from build123d import *

# Parameters (mm, degrees)
BASE_EXTRUDE_DEPTH = 3.048
SKETCH4_R          = 3.2385
REARRIB_DEPTH      = 3.048


with BuildPart() as part:
    # Sketch2 → Base-Extrude (new body)
    with BuildSketch(Plane(origin=(0, 0, 0), x_dir=(1, 0, 0), z_dir=(0, 1, 0))):
        with BuildLine():
            Line((0, 13.97), (7.747, 13.97))
            Line((7.747, 13.97), (7.747, 9.652))
            ThreePointArc((7.747, 9.652), (11.176, 6.223), (14.605, 9.652))
            Line((14.605, 9.652), (14.605, 13.97))
            Line((14.605, 13.97), (16.637, 13.97))
            ThreePointArc((16.637, 13.97), (19.061669153, 12.965669153), (20.066, 10.541))
            Line((20.066, 10.541), (20.066, -10.541))
            ThreePointArc((20.066, -10.541), (19.061669153, -12.965669153), (16.637, -13.97))
            Line((16.637, -13.97), (14.605, -13.97))
            Line((14.605, -13.97), (14.605, -9.398))
            ThreePointArc((14.605, -9.398), (11.176, -5.969), (7.747, -9.398))
            Line((7.747, -9.398), (7.747, -13.97))
            Line((7.747, -13.97), (0, -13.97))
            Line((0, -13.97), (0, 13.97))
        make_face()
    extrude(amount=BASE_EXTRUDE_DEPTH)

    # Sketch4 → RearRib (add)
    with BuildSketch(Plane.ZY):
        with BuildLine():
            Line((13.97, 22.352), (13.97, 0))
            Line((13.97, 0), (-13.97, 0))
            Line((-13.97, 0), (-13.97, 6.35))
            Line((-13.97, 6.35), (-0.465269586, 26.70511583))
            ThreePointArc((-0.465269586, 26.70511583), (8.369371866, 29.890677361), (13.97, 22.352))
        make_face()
        with Locations((6.096, 22.352)):
            Circle(SKETCH4_R, mode=Mode.SUBTRACT)
    extrude(amount=-REARRIB_DEPTH)


solid = part.part
Read the model definition and answer for the solid it produces. Units are mm, in the model's axes. A direction names the side the tool comes from. Round coordinates to 2 decimals unless told otherwise and drop trailing zeros. Write each loop counter-clockwise with the first axis right and the second up, starting at its lowest first coordinate (ties: lowest second). Pieces come first, ordered by that corner, then holes. Notation, with made-up numbers: (11, -10) - (51, -10) arc R15 ccw to (51, 16) - close; hole circle Ø3 at (-13, 83). An arc over 180 degrees is marked (long way). One line per question, with ' | ' between items. Start each with the question number.
1. Section A-A (x = 2) is taken. Determine the outline of the cut face in (y, z), and give its area (3 significant figures).
2. Find the intervals of material crossed by probe 1 along Y at (x, z) = (11.5, -2); probe 2 along Z at (x, y) = (2.5, 22), in increasing order. Write a range as [from, to].
3. Section D-D (x = 5) is taken. Determine the outline of the cut face in (y, z), and give its area (3 significant figures).
4. Section C-C (z = 10) is taken. Determine the outline of the cut face in (x, y) (3 decimals).
5. Section B-B (y = 20.5) is taken. Determine the outline of the cut face in (x, z), and give its area (3 significant figures).
6. For a pull along X with two mould halves and no side action, classify faces 1 (the face through (16, 2, 13.97)), 2 (the face through (11.101, 1.503, -6.224)), 3 (the face through (11.25, 1.5, 5.97)), 4 (the face through (19.035, 1.503, -12.992)) as +X half, -X half, draft (parallel to the pull), parting line (faces both ways), or undercut.
7. Each of these flat-tipped pins is pushed along its axis until it touches: pin 1 (1.5 mm diameter, centred on y = 8, z = 8, fed in from +X); pin 2 (1 mm diameter, centred on x = 8, z = 10.5, fed in from +Y); pin 3 (1 mm diameter, centred on x = 12.5, z = -9.5, fed in from -Y); pin 4 (3.5 mm diameter, centred on y = 1, z = 10.5, fed in from -X). Where does it stop, or does it pass through?
8. For faces 5 (the face through (1.5, 19.19, 5.39)), 6 (the face through (7.747, 2, 12)), 7 (the face through (12, 3.048, 0)), 8 (the face through (7.747, 2, -12)), determine the directions among +Z, -Z, +X, -X, +Y, -Y from which every point of the face is accessible in a straight line to the end or side of a thin tool.
Filled in:
1) outline: (0, -13.97) - (6.35, -13.97) - (26.71, -0.47) arc R7.87 ccw to (22.35, 13.97) - (0, 13.97) - close; hole circle Ø6.48 at (22.35, 6.1) | area: 606 mm²
2) probe 1: [0, 3.05] | probe 2: [-3.59, 2.88], [9.32, 13.97]
3) outline: (0, -13.97) - (3.05, -13.97) - (3.05, 13.97) - (0, 13.97) - close | area: 85.2 mm²
4) outline: (0, 0) - (7.747, 0) - (7.747, 3.048) - (3.048, 3.048) - (3.048, 29.19) - (0, 29.19) - close; (14.605, 0) - (20.066, 0) - (20.066, 3.048) - (14.605, 3.048) - close
5) outline: (0, -4.58) - (3.05, -4.58) - (3.05, 3.44) - (0, 3.44) - close; (0, 8.75) - (3.05, 8.75) - (3.05, 13.97) - (0, 13.97) - close | area: 40.4 mm²
6) face 1: draft | face 2: undercut | face 3: undercut | face 4: +X half
7) pin 1: x = 3.05 | pin 2: y = 3.05 | pin 3: through | pin 4: x = 0
8) face 5: +X, -X | face 6: +Z, +Y, -Y | face 7: +Z, -Z, +X, +Y | face 8: -Z, +Y, -Y
